Could you check a few things on this model? Use its own coordinates, in mm. A direction names the side the tool comes from. Coordinates: 2 decimals unless noted, no trailing zeros. Loops run counter-clockwise (first coordinate to the right, second up) from the corner with the lowest first, then second, coordinate; pieces in that order, holes last. Notation, with made-up numbers: (-35.75, -2) -> (-31.75, -2) arc R4 cw to (-31.75, 5) -> close; hole circle Ø7 at (17.25, 0). An arc over 180 degrees is marked (long way). One line per question, with ' | ' between items.
```python
from build123d import *

# Parameters (mm, degrees)
IMPORTED_BODY_2_1_OUTLINE_R = 2.25
IMPORTED_BODY_2_1_DEPTH     = 12
SKETCH_2_W                  = 124
SKETCH_2_H                  = 100
CUT_EXTRUDE_1_DEPTH         = 12


# Read off the part's stored shape, not the designer's step: 基体零件-零件2-1
with BuildPart() as part:
    # 基体零件-零件2-1 outline → 基体零件-零件2-1 (new body)
    with BuildSketch(Plane(origin=(0, 0, 0), x_dir=(1, 0, 0), z_dir=(0, 1, 0))):
        Polygon((0, -150), (0, -140), (3, -140), (3, -110), (0, -110), (0, -90), (3, -90), (3, -60), (0, -60), (0, -40), (3, -40), (3, -10), (0, -10), (0, 0), (-118, 0), (-118, -10), (-121, -10), (-121, -40), (-118, -40), (-118, -60), (-121, -60), (-121, -90), (-118, -90), (-118, -110), (-121, -110), (-121, -140), (-118, -140), (-118, -150), align=None)
        with Locations((-90.5, -130)):
            Circle(IMPORTED_BODY_2_1_OUTLINE_R, mode=Mode.SUBTRACT)
        with Locations((-81.5, -130)):
            Circle(IMPORTED_BODY_2_1_OUTLINE_R, mode=Mode.SUBTRACT)
        with Locations((-72.5, -130)):
            Circle(IMPORTED_BODY_2_1_OUTLINE_R, mode=Mode.SUBTRACT)
        with Locations((-63.5, -130)):
            Circle(IMPORTED_BODY_2_1_OUTLINE_R, mode=Mode.SUBTRACT)
        with Locations((-54.5, -130)):
            Circle(IMPORTED_BODY_2_1_OUTLINE_R, mode=Mode.SUBTRACT)
        with Locations((-45.5, -130)):
            Circle(IMPORTED_BODY_2_1_OUTLINE_R, mode=Mode.SUBTRACT)
        with Locations((-36.5, -130)):
            Circle(IMPORTED_BODY_2_1_OUTLINE_R, mode=Mode.SUBTRACT)
        with Locations((-27.5, -130)):
            Circle(IMPORTED_BODY_2_1_OUTLINE_R, mode=Mode.SUBTRACT)
    extrude(amount=IMPORTED_BODY_2_1_DEPTH)

    # 草图2 → 切除-拉伸1 (cut)
    with BuildSketch(Plane(origin=(0, 12, 0), x_dir=(1, 0, 0), z_dir=(0, 1, 0))):
        with Locations((-59, -50)):
            Rectangle(SKETCH_2_W, SKETCH_2_H)
    extrude(amount=-CUT_EXTRUDE_1_DEPTH, mode=Mode.SUBTRACT)


solid = part.part
```
Q1. Imagine slicing it at D-D on z = 141.5. Write out the boundary of the cut face in (x, y), plus the area to 3 significant figures.
Values follow:
outline: (-118, 0) -> (0, 0) -> (0, 12) -> (-118, 12) -> close | area: 1,420 mm2
Q2. For faces 1 (the face through (0, 6, 145)), 2 (the face through (-120, 6, 140)), 3 (the face through (2, 6, 110)), which set-ups out of +Z, -Z, +X, -X, +Y, -Y let a thin tool reach every point of the face, with its end or its side?
Values follow:
face 1: +Z, +X, +Y, -Y | face 2: +Z, -X, +Y, -Y | face 3: -Z, +X, +Y, -Y
Q3. Please list where these lines run through material, in increasing order: L1, parallel to Z at x = -81.5, y = 3; L2, parallel to X at y = 8.75, z = 146; L3, parallel to Z at x = -56.5, y = 5. Write a range as [from, to].
Values follow:
L1: z = [100, 127.75], [132.25, 150] | L2: x = [-118, 0] | L3: z = [100, 128.97], [131.03, 150]
Q4. We'd pull the mould along Z, two halves only. Please class faces 4 (the face through (-60, 6, 150)), 5 (the face through (-79.42, 5.92, 130.86)), 6 (the face through (3, 6, 125)): released by +Z, released by -Z, zero draft, split by the parting line, or undercut.
Values follow:
face 4: released by +Z | face 5: undercut | face 6: zero draft
Q5. Imagine slicing it at A-A on x = -54.5. Write out the boundary of the cut face in (y, z), plus the area to 3 significant figures.
Values follow:
outline: (0, 100) -> (12, 100) -> (12, 127.75) -> (0, 127.75) -> close; (0, 132.25) -> (12, 132.25) -> (12, 150) -> (0, 150) -> close | area: 546 mm2
Q6. For pin 1 (0.9 mm diameter, centred on x = -120, y = 7.5, fed in from -Z); pin 2 (6 mm diameter, centred on x = -36.5, z = 130, fed in from -Y); pin 3 (3.5 mm diameter, centred on x = -27.5, z = 130, fed in from +Y); pin 4 (5 mm diameter, centred on y = 7, z = 146, fed in from -X), each with a flat end and sliding along its axis, tell me the tip position at first contact or that it passes through.
Values follow:
pin 1: stops at z = 110 | pin 2: stops at y = 0 | pin 3: passes through | pin 4: stops at x = -118
Q7. Imagine slicing it at B-B on y = 2.5. Give the number of separate pieces and of enclosed holes in the cut face, plus the area to 3 significant figures.
Values follow:
separate pieces: 1 | enclosed holes: 8 | area: 5,950 mm2
Q8. Imagine slicing it at C-C on x = -28. Write out the boundary of the cut face in (y, z).
Values follow:
outline: (0, 100) -> (12, 100) -> (12, 127.81) -> (0, 127.81) -> close; (0, 132.19) -> (12, 132.19) -> (12, 150) -> (0, 150) -> close
